from build123d import *

# Parameters (mm, degrees)
SKETCH001_R     = 28.5
PAD_DEPTH       = 5
SKETCH002_R     = 37.875
PAD001_DEPTH    = 5
CHAMFER_SIZE    = 1
CHAMFER001_SIZE = 0.75


with BuildPart() as part:
    # Sketch001 → Pad (new body)
    with BuildSketch(Plane.XZ.offset(29)):
        Circle(SKETCH001_R)
    extrude(amount=PAD_DEPTH)

    # Sketch002 (on Face3 of Pad) → Pad001 (join)
    with BuildSketch(Plane.XZ.offset(34)):
        Circle(SKETCH002_R)
    extrude(amount=PAD001_DEPTH)

    # Chamfer
    chamfer_edges = [part.edges().sort_by_distance(p)[0] for p in [
        (-37.875, -39, 0),
        (-37.875, -34, 0),
    ]]
    chamfer(chamfer_edges, length=CHAMFER_SIZE)

    # Chamfer001
    chamfer001_edges = [part.edges().sort_by_distance(p)[0] for p in [
        (-28.5, -29, 0),
    ]]
    chamfer(chamfer001_edges, length=CHAMFER001_SIZE)


solid = part.part
Verification items for the finished model (mm, model axes). A direction names the side the tool comes from. Coordinates: 2 decimals unless noted, no trailing zeros. Write each loop counter-clockwise with the first axis right and the second up, starting at its lowest first coordinate (ties: lowest second). Pieces come first, ordered by that corner, then holes. Notation, with made-up numbers: M 52,31 L 97,31 A16 cw 97,57 Z; hole C 29.25,23 d2. An arc over 180 degrees is marked long. Use CSV: the item, a comma, the result in double quotes.
Q1. Section check C-C, the plane y = -36. Enter the section's corners in (x, z) (3 decimals), and give its area (3 significant figures).
Computed values:
outline,"C 0,0 d75.75"
area,"4,510 mm²"
Q2. Thickness scan on line 1 along Y through (x, z) = (-6, -34); line 2 along Z through (x, y) = (18.5, -37); line 3 along X through (y, z) = (-32.5, 18). Record the ranges inside material, lowest first. Write a range as [from, to].
Computed values:
line 1,"[-39, -34]"
line 2,"[-33.05, 33.05]"
line 3,"[-22.1, 22.1]"
Q3. Section check D-D, the plane y = -32. Enter the section's corners in (x, z).
Computed values:
outline,"C 0,0 d57"
Q4. Set-up check for faces 1 (the cylindrical face through (26.327, -31.845, -10.916)), 2 (the flat face through (0, -29, 0)): record each of +Z, -Z, +X, -X, +Y, -Y from which the full face is reachable in a straight line by a thin tool's end or side.
Computed values:
face 1,"+Y"
face 2,"+Z, -Z, +X, -X, +Y"
Q5. Section check B-B, the plane x = 0. Enter the section's corners in (y, z) (3 decimals).
Computed values:
outline,"M -39,-36.875 L -38,-37.875 L -35,-37.875 L -34,-36.875 L -34,-28.5 L -29.75,-28.5 L -29,-27.75 L -29,27.75 L -29.75,28.5 L -34,28.5 L -34,36.875 L -35,37.875 L -38,37.875 L -39,36.875 Z"
Q6. Go/stop test with flat-tipped pins: P1, Ø4, axis at y = -37.5, z = -9.5, coming from the +X side (3 decimals); P2, Ø6, axis at y = -35.5, z = 11, coming from the -X side; P3, Ø3, axis at x = 19, z = 27.5, coming from the +Y side. Record where each tip stops, or that it passes through.
Computed values:
P1,"x = 37.125"
P2,"x = -37.02"
P3,"y = -34"
Q7. Section check A-A, the plane z = 0. Enter the section's corners in (x, y) (3 decimals), and give its area (3 significant figures).
Computed values:
outline,"M -37.875,-38 L -36.875,-39 L 36.875,-39 L 37.875,-38 L 37.875,-35 L 36.875,-34 L 28.5,-34 L 28.5,-29.75 L 27.75,-29 L -27.75,-29 L -28.5,-29.75 L -28.5,-34 L -36.875,-34 L -37.875,-35 Z"
area,"661 mm²"
